The listing builds one solid part. Answer for the finished solid, in the listing's coordinates (mm). A direction names the side the tool comes from. Round coordinates to 2 decimals unless told otherwise and drop trailing zeros. Write each loop counter-clockwise with the first axis right and the second up, starting at its lowest first coordinate (ties: lowest second). Pieces come first, ordered by that corner, then holes.
from build123d import *

# Parameters (mm, degrees)
F0_R     = 1.6132793462
F0_R_2   = 1.6452292319
F1_DEPTH = 5
F4_DEPTH = 52
F5_W     = 5.1189595833
F5_H     = 18.4771826025
F6_DEPTH = 78.0283830646
F7_R     = 4.99999
F8_R     = 2.8294209196
F8_R_2   = 2.8212759524
F8_R_3   = 7.3886605842
F9_DEPTH = 25


# Not quite as in the source:
# - a fillet or chamfer is up to 0.001 mm smaller than in the source, because OpenCascade refuses the exact size


with BuildPart() as f1:
    # F0 (on Front) → F1 (new body)
    with BuildSketch(Plane.XZ):
        with BuildLine():
            Line((-40.6402352101, -8.6803976446), (45.1620352523, -8.6803976446))
            ThreePointArc((45.1620352523, -8.6803976446), (52.5455844959, -11.7387638798), (49.4872182608, -4.3552146362))
            Line((49.4872182608, -4.3552146362), (49.4872182608, -4.395077005))
            Line((49.4872182608, -4.395077005), (28.2908082008, -4.395077005))
            Line((28.2908082008, -4.395077005), (28.2908082008, 21.208807826))
            Line((28.2908082008, 21.208807826), (-23.8502826542, 21.208807826))
            Line((-23.8502826542, 21.208807826), (-23.8502826542, -4.395077005))
            Line((-23.8502826542, -4.395077005), (-44.8338091373, -4.395077005))
            Line((-44.8338091373, -4.395077005), (-44.8338091373, -4.4868237174))
            ThreePointArc((-44.8338091373, -4.4868237174), (-47.7991136987, -11.645702206), (-40.6402352101, -8.6803976446))
        make_face()
        with Locations((-44.8338091373, -8.6803976446)):
            Circle(F0_R, mode=Mode.SUBTRACT)
        with Locations((49.4872182608, -8.6803976446)):
            Circle(F0_R_2, mode=Mode.SUBTRACT)
    extrude(amount=F1_DEPTH)

    # F3 (on offset) → F4 (join)
    with BuildSketch(Plane.YZ.offset(29)):
        Polygon((14.035618864, 23.0911467224), (-5.0185876898, -4.3173860759), (0, -4.3494757265), (18.4650830925, 23.0911467224), align=None)
    extrude(amount=-F4_DEPTH)

    # F5 (on offset) → F6 (cut, through all)
    with BuildSketch(Plane.YZ.offset(29)):
        with Locations((-2.5594797917, 12.1628475608)):
            Rectangle(F5_W, F5_H)
    extrude(amount=-F6_DEPTH, mode=Mode.SUBTRACT)

    # F7 (radius 5 in the source; OpenCascade refuses exactly that, so slightly less here)
    f7_edges = [f1.edges().sort_by_distance(p)[0] for p in [
        (-23, 16.250351, 23.091147),
        (29, 16.250351, 23.091147),
        (2.220263, -5, 2.924256),
    ]]
    fillet(f7_edges, radius=F7_R)

    # F8 (on face) → F9 (cut)
    with BuildSketch(Plane(origin=(0, 0, 0), x_dir=(-1, 0, 0), z_dir=(0, 1, 0))):
        with Locations((-22.5741807371, -4.3494757265)):
            Circle(F8_R)
        with Locations((16.9429704547, -4.3494757265)):
            Circle(F8_R_2)
        with Locations((-2.2609000211, -11.7509029806)):
            Circle(F8_R_3)
    extrude(amount=-F9_DEPTH, mode=Mode.SUBTRACT)


solid = f1.part
1. Section C-C on z = 1 is taken. Determine the outline of the cut face in (x, y).
Geometry says:
outline: (-23.85, -3.94) - (28.29, -3.94) - (28.29, -1.32) - (29, -1.32) - (29, 3.6) - (-23, 3.6) - (-23, 0) - (-23.85, 0) - close
2. Section A-A on y = -2.25 is taken. Give the number of separate pieces and of enclosed holes in the cut face, plus the area to 3 significant figures.
Geometry says:
separate pieces: 1
enclosed holes: 4
area: 738 mm2
3. A tool of negligible diameter and unlimited length cuts with its end or side. For faces 1 (the face through (27, -2, -8.68)), 2 (the face through (19.875, -2.474, -3.5)), 3 (the face through (29, 5, 6)), 4 (the face through (-34, -2, -4.395)), 5 (the face through (-47.895, -2.465, -11.546)), from which of +Z, -Z, +X, -X, +Y, -Y can it reach the whole face along a straight path? Write none if from no direction.
Geometry says:
face 1: -Z, +Y, -Y
face 2: -Y
face 3: +Z, +X, +Y, -Y
face 4: +Z, -X, +Y, -Y
face 5: +Y, -Y
4. Given pin 1 (2.5 mm diameter, centred on x = -37, y = -2.5, fed in from +Z); pin 2 (5.5 mm diameter, centred on x = -23.5, y = -1.5, fed in from -Z); pin 3 (5 mm diameter, centred on x = 23.5, z = 5.5, fed in from +Y), each flat-ended and moving along its own axis, determine where each tip first touches the part or whether it passes through.
Geometry says:
pin 1: stops at z = -4.4
pin 2: stops at z = -8.68
pin 3: stops at y = 8.31
5. Section B-B on x = 42.5 is taken. Determine the outline of the cut face in (y, z), plus the area to 3 significant figures.
Geometry says:
outline: (-5, -8.68) - (0, -8.68) - (0, -4.4) - (-5, -4.4) - close
area: 21.4 mm2
6. Section D-D on y = 3 is taken. Determine the outline of the cut face in (x, z).
Geometry says:
outline: (-23, 0.11) - (29, 0.11) - (29, 7.22) - (-23, 7.22) - close
7. For a pull along X with two mould halves and no side action, classify faces 6 (the face through (-23, 7, 9)), 7 (the face through (28.291, -3, 0)), 8 (the face through (-19.634, -2.474, -3.502)) as released by +X, released by -X, zero draft, split by the parting line, or undercut.
Geometry says:
face 6: released by -X
face 7: released by +X
face 8: undercut
8. Straight lines are drawn through the part: line 1 along X through (y, z) = (9.5, 11); line 2 along X through (y, z) = (-2.5, -3.5); line 3 along Z through (x, y) = (-34, -1.75). For each, find the intervals that lie inside material, in ascending order.
Geometry says:
line 1: x = -23 to 29
line 2: x = -23.85 to -19.63, -14.25 to 19.88, 25.27 to 29
line 3: z = -8.68 to -4.4
